The model under review builds one solid part; all positions refer to its coordinate system, in mm. Face numbers are marked on the shaded views. A direction names the side the tool comes from. Coordinates: 2 decimals unless noted, no trailing zeros. Write each loop counter-clockwise with the first axis right and the second up, starting at its lowest first coordinate (ties: lowest second). Pieces come first, ordered by that corner, then holes. Notation, with made-up numbers: (14, 0) - (52, 0) arc R12 ccw to (52, 20) - close; hole circle Ø8 at (87.25, 30). An arc over 180 degrees is marked (long way). Put each result on its own line as item: value.
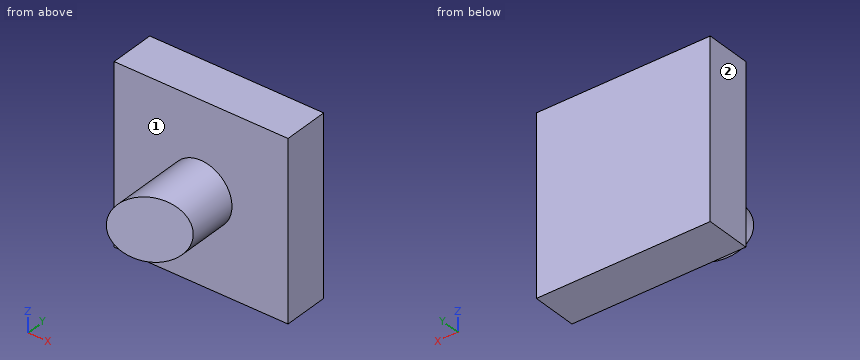
from build123d import *

# Parameters (mm, degrees)
F0_W     = 97.346954
F0_H     = 98.902032
F1_DEPTH = 25.4
F2_R     = 17.286397
F3_DEPTH = 50.8
F5_DEPTH = 35.814


with BuildPart() as f1:
    # F0 (on Front) → F1 (new body)
    with BuildSketch(Plane.XZ):
        Rectangle(F0_W, F0_H)
    extrude(amount=F1_DEPTH)

    # F2 (on face) → F3 (join)
    with BuildSketch(Plane.XZ.offset(25.4)):
        Circle(F2_R)
    extrude(amount=F3_DEPTH)

    # F4 (on Top) → F5 (cut, symmetric)
    with BuildSketch(Plane.XY):
        Polygon((48.688538, -36.72133), (-35.245914, -80.327898), (48.688538, -80.327898), align=None)
    extrude(amount=F5_DEPTH, both=True, mode=Mode.SUBTRACT)


solid = f1.part
1. Consider section C-C on y = -38. State the section outline as (x, z) points.
Determined:
outline: circle Ø34.57 at (0, 0)
2. Machinability: for the marked faces 1 and 2, which of the approach directions +Z, -Z, +X, -X, +Y, -Y give a long, thin tool a straight path to every point of the face, cutting with its end or side? Answer none if there is none.
Determined:
face 1: -Y
face 2: +Z, -Z, -X, +Y, -Y
3. Consider section A-A on z = 0. State the section outline as (x, y) points, plus the area to 3 significant figures.
Determined:
outline: (-48.67, -25.4) - (-17.29, -25.4) - (-17.29, -71) - (17.29, -53.04) - (17.29, -25.4) - (48.67, -25.4) - (48.67, 0) - (-48.67, 0) - close
area: 3,740 mm^2
4. For pin 1 Ø8 at (x, z) = (31, -6.5) entering from +Y; pin 2 Ø8 at (y, z) = (-41, 24) entering from +X; pin 3 Ø3 at (y, z) = (-34.5, 15.5) entering from -X; pin 4 Ø4 at (x, z) = (-6.5, -4.5) entering from -Y, all flat-tipped, find the tip position at first contact; note any pin that passes through.
Determined:
pin 1: stops at y = 0
pin 2: passes through
pin 3: stops at x = -10.14
pin 4: stops at y = -66.43
5. Consider section B-B on x = 43. State the section outline as (y, z) points.
Determined:
outline: (-25.4, -49.45) - (0, -49.45) - (0, 49.45) - (-25.4, 49.45) - close
6. Consider section D-D on x = -7. State the section outline as (y, z) points.
Determined:
outline: (-65.65, -15.81) - (-25.4, -15.81) - (-25.4, -49.45) - (0, -49.45) - (0, 49.45) - (-25.4, 49.45) - (-25.4, 15.81) - (-65.65, 15.81) - close
7. To check wall thickness, follow probe 1 along Y at (x, z) = (24.5, 24); probe 2 along X at (y, z) = (-26, 2); probe 3 along Z at (x, y) = (-9.5, -52.5). State the ranges of each line that lie inside material, in increasing order.
Determined:
probe 1: y = -25.4 to 0
probe 2: x = -17.17 to 17.17
probe 3: z = -14.44 to 14.44
